```python
from build123d import *

# Parameters (mm, degrees)
BOSS_EXTRUDE3_DEPTH = 15.24
SKETCH6_R           = 3.175
CUT_EXTRUDE2_DEPTH  = 16.24
CUT_EXTRUDE6_REACH  = 17.24
SKETCH53_R          = 2.413
FILLET1_R           = 3.81
SKETCH57_R          = 3.96875
CUT_EXTRUDE8_DEPTH  = 12.7
SKETCH55_R          = 3.96875
CUT_EXTRUDE9_DEPTH  = 12.7
CIRPATTERN2_COUNT   = 4
SKETCH58_R          = 3.96875
CUT_EXTRUDE10_DEPTH = 12.7
CIRPATTERN3_COUNT   = 4


with BuildPart() as part:
    # Sketch5 → Boss-Extrude3 (new body)
    with BuildSketch(Plane(origin=(0, 0, 0), x_dir=(1, 0, 0), z_dir=(0, 1, 0))):
        with BuildLine():
            Line((-11.833206742, -44.162128778), (-88.108068982, -120.436991017))
            ThreePointArc((-88.108068982, -120.436991017), (-105.518009423, -105.518009423), (-120.436991017, -88.108068982))
            Line((-120.436991017, -88.108068982), (-44.162128778, -11.833206742))
            ThreePointArc((-44.162128778, -11.833206742), (-45.72, 0), (-44.162128778, 11.833206742))
            Line((-44.162128778, 11.833206742), (-120.436991017, 88.108068982))
            ThreePointArc((-120.436991017, 88.108068982), (-105.518009423, 105.518009423), (-88.108068982, 120.436991017))
            Line((-88.108068982, 120.436991017), (-11.833206742, 44.162128778))
            ThreePointArc((-11.833206742, 44.162128778), (0, 45.72), (11.833206742, 44.162128778))
            Line((11.833206742, 44.162128778), (88.108068982, 120.436991017))
            ThreePointArc((88.108068982, 120.436991017), (105.518009423, 105.518009423), (120.436991017, 88.108068982))
            Line((120.436991017, 88.108068982), (44.162128778, 11.833206742))
            ThreePointArc((44.162128778, 11.833206742), (45.72, 0), (44.162128778, -11.833206742))
            Line((44.162128778, -11.833206742), (120.436991017, -88.108068982))
            ThreePointArc((120.436991017, -88.108068982), (105.518009423, -105.518009423), (88.108068982, -120.436991017))
            Line((88.108068982, -120.436991017), (11.833206742, -44.162128778))
            ThreePointArc((11.833206742, -44.162128778), (0, -45.72), (-11.833206742, -44.162128778))
        make_face()
    extrude(amount=BOSS_EXTRUDE3_DEPTH)

    # Sketch6 → Cut-Extrude2 (cut, through all)
    with BuildSketch(Plane(origin=(0, 15.24, 0), x_dir=(1, 0, 0), z_dir=(0, 1, 0))):
        with Locations((-74.536125805, -94.292689271)):
            Circle(SKETCH6_R)
        with Locations((-94.292689271, -74.536125805)):
            Circle(SKETCH6_R)
        with Locations((94.292689271, -74.536125805)):
            Circle(SKETCH6_R)
        with Locations((74.536125805, -94.292689271)):
            Circle(SKETCH6_R)
        with Locations((94.292689271, 74.536125805)):
            Circle(SKETCH6_R)
        with Locations((74.536125805, 94.292689271)):
            Circle(SKETCH6_R)
        with Locations((-94.292689271, 74.536125805)):
            Circle(SKETCH6_R)
        with Locations((-74.536125805, 94.292689271)):
            Circle(SKETCH6_R)
    extrude(amount=-CUT_EXTRUDE2_DEPTH, mode=Mode.SUBTRACT)

    # Sketch53 → Cut-Extrude6 (cut, up to next)
    with BuildSketch(Plane(origin=(0, 15.24, 0), x_dir=(1, 0, 0), z_dir=(0, 1, 0)), mode=Mode.PRIVATE) as cut_extrude6_sk1:
        with Locations((-88.455522793, -101.027881362)):
            Circle(SKETCH53_R)
    cut_extrude6_tool1 = extrude(cut_extrude6_sk1.sketch, amount=-CUT_EXTRUDE6_REACH, mode=Mode.PRIVATE) & part.part
    add(cut_extrude6_tool1.solids().sort_by_distance((-88.455523, 15.24, 101.027881))[0], mode=Mode.SUBTRACT)
    # Sketch53 → Cut-Extrude6 (cut, up to next)
    with BuildSketch(Plane(origin=(0, 15.24, 0), x_dir=(1, 0, 0), z_dir=(0, 1, 0)), mode=Mode.PRIVATE) as cut_extrude6_sk2:
        with Locations((-61.514754429, -74.087112999)):
            Circle(SKETCH53_R)
    cut_extrude6_tool2 = extrude(cut_extrude6_sk2.sketch, amount=-CUT_EXTRUDE6_REACH, mode=Mode.PRIVATE) & part.part
    add(cut_extrude6_tool2.solids().sort_by_distance((-61.514754, 15.24, 74.087113))[0], mode=Mode.SUBTRACT)
    # Sketch53 → Cut-Extrude6 (cut, up to next)
    with BuildSketch(Plane(origin=(0, 15.24, 0), x_dir=(1, 0, 0), z_dir=(0, 1, 0)), mode=Mode.PRIVATE) as cut_extrude6_sk3:
        with Locations((-101.925906974, -87.55749718)):
            Circle(SKETCH53_R)
    cut_extrude6_tool3 = extrude(cut_extrude6_sk3.sketch, amount=-CUT_EXTRUDE6_REACH, mode=Mode.PRIVATE) & part.part
    add(cut_extrude6_tool3.solids().sort_by_distance((-101.925907, 15.24, 87.557497))[0], mode=Mode.SUBTRACT)
    # Sketch53 → Cut-Extrude6 (cut, up to next)
    with BuildSketch(Plane(origin=(0, 15.24, 0), x_dir=(1, 0, 0), z_dir=(0, 1, 0)), mode=Mode.PRIVATE) as cut_extrude6_sk4:
        with Locations((-74.985138611, -60.616728817)):
            Circle(SKETCH53_R)
    cut_extrude6_tool4 = extrude(cut_extrude6_sk4.sketch, amount=-CUT_EXTRUDE6_REACH, mode=Mode.PRIVATE) & part.part
    add(cut_extrude6_tool4.solids().sort_by_distance((-74.985139, 15.24, 60.616729))[0], mode=Mode.SUBTRACT)

    # Fillet1
    fillet1_edges = [part.edges().sort_by_distance(p)[0] for p in [
        (-44.162128778, 7.62, 11.833206742),
        (-44.162128778, 7.62, -11.833206742),
        (-11.833206742, 7.62, -44.162128778),
        (11.833206742, 7.62, -44.162128778),
        (44.162128778, 7.62, -11.833206742),
        (44.162128778, 7.62, 11.833206742),
        (11.833206742, 7.62, 44.162128778),
        (-11.833206742, 7.62, 44.162128778),
    ]]
    fillet(fillet1_edges, radius=FILLET1_R)

    # Sketch57 → Cut-Extrude8 (cut)
    with BuildSketch(Plane(origin=(-114.312982024, 0, 95.919981055), x_dir=(0.64278761, 0, 0.766044443), z_dir=(-0.766044443, 0, 0.64278761))):
        with Locations((0, 7.62)):
            Circle(SKETCH57_R)
    cut_extrude8 = extrude(amount=-CUT_EXTRUDE8_DEPTH, mode=Mode.SUBTRACT)

    # Sketch55 → Cut-Extrude9 (cut)
    with BuildSketch(Plane(origin=(-95.919981055, 0, 114.312982024), x_dir=(0.766044443, 0, 0.64278761), z_dir=(-0.64278761, 0, 0.766044443))):
        with Locations((0, 7.62)):
            Circle(SKETCH55_R)
    cut_extrude9 = extrude(amount=-CUT_EXTRUDE9_DEPTH, mode=Mode.SUBTRACT)

    # CirPattern2: Cut-Extrude8, Cut-Extrude9 ×4 about axis
    cirpattern2_axis = Axis((0, 0, 0), (0, 1, 0))
    for i in range(1, CIRPATTERN2_COUNT):
        add(cut_extrude8.rotate(cirpattern2_axis, i * 360 / CIRPATTERN2_COUNT), mode=Mode.SUBTRACT)
        add(cut_extrude9.rotate(cirpattern2_axis, i * 360 / CIRPATTERN2_COUNT), mode=Mode.SUBTRACT)

    # Sketch58 → Cut-Extrude10 (cut)
    with BuildSketch(Plane(origin=(-105.518009423, 0, 105.518009423), x_dir=(0.707106781, 0, 0.707106781), z_dir=(-0.707106781, 0, 0.707106781))):
        with Locations((0, 7.62)):
            Circle(SKETCH58_R)
    cut_extrude10 = extrude(amount=-CUT_EXTRUDE10_DEPTH, mode=Mode.SUBTRACT)

    # CirPattern3: Cut-Extrude10 ×4 about axis
    cirpattern3_axis = Axis((0, 0, 0), (0, 1, 0))
    for i in range(1, CIRPATTERN3_COUNT):
        add(cut_extrude10.rotate(cirpattern3_axis, i * 360 / CIRPATTERN3_COUNT), mode=Mode.SUBTRACT)


solid = part.part
```
Geometry check sheet. Reference: the model listing, model coordinates, mm. A direction names the side the tool comes from. Coordinates: 2 decimals unless noted, no trailing zeros. Loops run counter-clockwise (first coordinate to the right, second up) from the corner with the lowest first, then second, coordinate; pieces in that order, holes last.
Item 1: Sectioned sample at A-A, the plane x = -54.5. Record the boundary of the cut face in (y, z), then the cut area to 3 significant figures.
Item 2: Access from +Z, -Z, +X, -X, +Y, -Y to the whole of each face (thin tool, end or side, straight path). Record for faces 5 (the face through (-87.714, 7.676, -104.62)), 6 (the face through (-96.633, 7.727, -76.682)), 7 (the face through (-50.2, 7.51, 82.53)).
Item 3: Go/stop test with flat-tipped pins: pin 1 Ø8 at (x, y) = (-8.5, 5.5) entering from +Z; pin 2 Ø6 at (y, z) = (10, -3.5) entering from -X; pin 3 Ø8.5 at (x, z) = (94.29, -74.54) entering from -Y; pin 4 Ø1.5 at (x, y) = (63.5, 2) entering from +Z. Record where each tip stops, or that it passes through.
Item 4: Sectioned sample at C-C, the plane z = 32. Record the boundary of the cut face in (x, y), then the cut area to 3 significant figures.
Item 5: Thickness scan on line 1 (Z direction, x = 97, y = 9.5); line 2 (X direction, y = 10.75, z = 110); line 3 (Z direction, x = -59.5, y = 5.75). Record the ranges inside material, lowest first.
Item 6: Sectioned sample at B-B, the plane x = 41. Record the boundary of the cut face in (y, z), then the cut area to 3 significant figures.
Item 7: Release check for a two-part mould opening along Z. For faces 1 (the face through (96.498, 7.676, 96.577)), 2 (the face through (-0.14, 7.51, -45.72)), 3 (the face through (2, 0, -2)), 4 (the face through (-83.58, 7.51, 51.25)) record: released by +Z, released by -Z, zero draft, split by the parting line, or undercut.
Check result:
1. outline: (0, -86.83) - (15.24, -86.83) - (15.24, -22.17) - (0, -22.17) - close; (0, 22.17) - (15.24, 22.17) - (15.24, 86.83) - (0, 86.83) - close
1. area: 1,970 mm2
2. face 5: none
2. face 6: +Y, -Y
2. face 7: +Z, +Y, -Y
3. pin 1: stops at z = 45.5
3. pin 2: stops at x = -45.72
3. pin 3: stops at y = 0
3. pin 4: stops at z = 96.58
4. outline: (-64.33, 0) - (64.33, 0) - (64.33, 15.24) - (-64.33, 15.24) - close
4. area: 1,960 mm2
5. line 1: z = -110.16 to -101.94, -96.08 to -76.19, -72.88 to -64.67, 64.67 to 72.88, 76.19 to 96.08, 101.94 to 110.16
5. line 2: x = -100.84 to -95.49, -89.12 to -77.67, 77.67 to 89.12, 95.49 to 100.84
5. line 3: z = -91.83 to -27.17, 27.17 to 72.76, 75.42 to 91.83
6. outline: (0, -73.33) - (15.24, -73.33) - (15.24, 73.33) - (0, 73.33) - close
6. area: 2,240 mm2
7. face 1: undercut
7. face 2: released by -Z
7. face 3: zero draft
7. face 4: undercut
